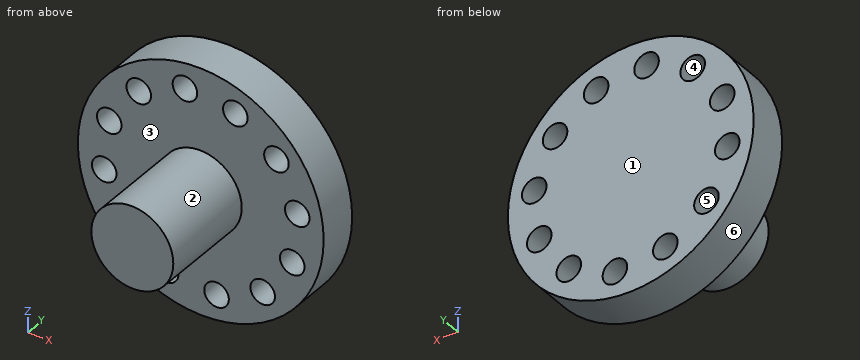
```python
from build123d import *

# Parameters (mm, degrees)
F0_R            = 15
F2_DEPTH        = 5
F1_R            = 1.5
F3_DEPTH        = 6
F3_COPIES_COUNT = 12
F4_R            = 5
F5_DEPTH        = 17


# Not quite as in the source:
# - a pattern or mirror of a feature is missing from the dataset's text; its kind, count and spacing are read off the source's solid


with BuildPart() as f2:
    # F0 (on Front) → F2 (new body)
    with BuildSketch(Plane.XZ):
        Circle(F0_R)
    extrude(amount=F2_DEPTH)

    # F1 (on face) → F3 (cut)
    with BuildSketch(Plane.XZ):
        with Locations((-7.5604245067, 9.2375520617)):
            Circle(F1_R)
    f3 = extrude(amount=F3_DEPTH, mode=Mode.SUBTRACT)

    # F3_copies: F3 ×12 about axis
    f3_copies_axis = Axis((0, 0, 0), (0, 1, 0))
    for i in range(1, F3_COPIES_COUNT):
        add(f3.rotate(f3_copies_axis, i * 360 / F3_COPIES_COUNT), mode=Mode.SUBTRACT)

    # F4 (on face) → F5 (join)
    with BuildSketch(Plane.XZ):
        Circle(F4_R)
    extrude(amount=F5_DEPTH)


solid = f2.part
```
The model under review builds one solid part; all positions refer to its coordinate system, in mm. Face numbers are marked on the shaded views. A direction names the side the tool comes from. Round coordinates to 2 decimals unless told otherwise and drop trailing zeros. Order: outer loops, then holes, each group sorted by start corner. A loop starts at its lowest first (then second) coordinate and runs counter-clockwise, first axis right, second up.
Item 1: Add section D-D, the plane z = -7. State the section outline as (x, y) points, and give its area (3 significant figures).
Working result:
outline: (-13.27, -5) - (-10.63, -5) - (-10.63, 0) - (-13.27, 0) - close; (-7.85, -5) - (13.27, -5) - (13.27, 0) - (-7.85, 0) - close
area: 119 mm2
Item 2: Add section C-C, the plane x = 0. State the section outline as (y, z) points, and give its area (3 significant figures).
Working result:
outline: (-17, -5) - (-5, -5) - (-5, -15) - (0, -15) - (0, 15) - (-5, 15) - (-5, 5) - (-17, 5) - close
area: 270 mm2
Item 3: For pin 1 (4 mm diameter, centred on x = 6.5, y = -10.5, fed in from -Z); pin 2 (4 mm diameter, centred on x = 7.56, z = -9.24, fed in from -Y); pin 3 (5 mm diameter, centred on y = -4, z = -9.5, fed in from -X), all flat-tipped, find the tip position at first contact; note any pin that passes through.
Working result:
pin 1: stops at z = -2.18
pin 2: stops at y = -5
pin 3: stops at x = -13.27
Item 4: Draft analysis for pull direction X (two halves, no side actions). For the marked faces 3, 4, 5 and 6, state which applies: released by +X, released by -X, zero draft, split by the parting line, or undercut.
Working result:
face 3: zero draft
face 4: undercut
face 5: undercut
face 6: split by the parting line
Item 5: Add section A-A, the plane x = -4.25. State the section outline as (y, z) points, and give its area (3 significant figures).
Working result:
outline: (-17, -2.63) - (-5, -2.63) - (-5, -9.67) - (0, -9.67) - (0, 14.39) - (-5, 14.39) - (-5, 2.63) - (-17, 2.63) - close; (-5, -14.39) - (0, -14.39) - (0, -12.67) - (-5, -12.67) - close
area: 192 mm2
Item 6: Add section B-B, the plane z = 0. State the section outline as (x, y) points.
Working result:
outline: (-15, -5) - (-5, -5) - (-5, -17) - (5, -17) - (5, -5) - (15, -5) - (15, 0) - (-15, 0) - close
Item 7: Machinability: for the marked faces 1 and 2, which of the approach directions +Z, -Z, +X, -X, +Y, -Y give a long, thin tool a straight path to every point of the face, cutting with its end or side? Answer none if there is none.
Working result:
face 1: +Z, -Z, +X, -X, +Y
face 2: -Y
Item 8: To check wall thickness, follow probe 1 along X at (y, z) = (-0.75, 3); probe 2 along Y at (x, z) = (9.75, 0.75); probe 3 along X at (y, z) = (-3, -10). State the ranges of each line that lie inside material, in increasing order.
Working result:
probe 1: x = -14.7 to -12.04, -10.29 to 10.73, 12.83 to 14.7
probe 2: y = -5 to 0
probe 3: x = -11.18 to -5.16, -3.28 to 6.27, 8.85 to 11.18
